Autodesk Inventor part; units mm, degrees
ref_plane "YZ Plane" through (0, 0, 0) normal (1, 0, 0) x (0, 1, 0)
ref_plane "XZ Plane" through (0, 0, 0) normal (0, 1, 0) x (-1, 0, 0)
ref_plane "XY Plane" through (0, 0, 0) normal (0, 0, 1) x (1, 0, 0)
sketch "Sketch1" plane through (0, 0, 0) normal (0, 0, 1) x (1, 0, 0)
  line L0 (68.58, 6.35) -> (68.58, 57.15)
  line L1 (68.58, 57.15) -> (0, 57.15)
  line L2 (0, 57.15) -> (0, 6.35)
  line L3 (40.64, 6.35) -> (40.64, 0)
  line L4 (27.94, 6.35) -> (27.94, 0)
  line L5 (27.94, 0) -> (40.64, 0)
  line L6 (27.94, 6.35) -> (18.8722, 6.35)
  line L7 (18.8722, 6.35) -> (18.8722, 0)
  line L8 (18.8722, 0) -> (6.1722, 0)
  line L9 (6.1722, 0) -> (6.1722, 6.35)
  line L10 (40.64, 6.35) -> (49.7078, 6.35)
  line L11 (49.7078, 6.35) -> (49.7078, 0)
  line L12 (49.7078, 0) -> (62.4078, 0)
  line L13 (62.4078, 0) -> (62.4078, 6.35)
  line L14 (6.1722, 0) -> (18.8722, 0)
  line L15 (27.94, 0) -> (40.64, 0)
  line L16 (49.7078, 0) -> (62.4078, 0)
  line L17 (27.94, 6.35) -> (18.8722, 6.35)
  line L18 (6.1722, 6.35) -> (0, 6.35)
  line L19 (40.64, 6.35) -> (49.7078, 6.35)
  line L20 (62.4078, 6.35) -> (68.58, 6.35)
  point P0 (0, 0)
  dimension "d0" = 68.58
  dimension "d1" = 50.8
extrude "Extrusion1" add sketch "Sketch1" against normal blind 6.35
sketch "Sketch2" plane through (0, 0, 0) normal (0, 0, 1) x (1, 0, 0)
  line L0 (0, 6.35) -> (6.1722, 6.35)
  line L1 (6.1722, 50.8) -> (6.1722, 57.15)
  line L2 (0, 57.15) -> (68.58, 57.15)
  line L3 (49.7078, 6.35) -> (40.64, 6.35)
  line L4 (40.64, 50.8) -> (40.64, 57.15)
  line L5 (18.8722, 0) -> (18.8722, 6.35)
  line L6 (18.8722, 50.8) -> (18.8722, 57.15)
  line L7 (27.94, 0) -> (27.94, 6.35)
  line L8 (27.94, 50.8) -> (27.94, 57.15)
  line L9 (49.7078, 50.8) -> (49.7078, 57.15)
  line L10 (68.58, 6.35) -> (62.4078, 6.35)
  line L11 (62.4078, 50.8) -> (62.4078, 57.15)
  line L12 (0, 57.15) -> (0, 50.8)
  line L13 (68.58, 57.15) -> (68.58, 6.35)
  line L14 (49.7078, 50.8) -> (62.4078, 50.8)
  line L15 (6.1722, 50.8) -> (18.8722, 50.8)
  line L16 (27.94, 50.8) -> (40.64, 50.8)
  line L17 (27.94, 57.15) -> (40.64, 57.15)
  point P0 (0, 0)
extrude "Extrusion2" cut sketch "Sketch2" against normal blind 6.35
properties part number "flat-no-recess"
Work out the finished part from the listing and answer in its coordinate system (mm). A direction names the side the tool comes from. Round coordinates to 2 decimals unless told otherwise and drop trailing zeros. Write each loop counter-clockwise with the first axis right and the second up, starting at its lowest first coordinate (ties: lowest second). Pieces come first, ordered by that corner, then holes. Notation, with made-up numbers: (75.25, 50.25) - (82.25, 50.25) arc R21 ccw to (82.25, 61.25) - close; hole circle Ø3 at (-6, -29.75). An arc over 180 degrees is marked (long way). Return JSON: item names as keys, results as strings. Group by question number.
Q1. For faces 4 (the flat face through (62.408, 54, -3)), 5 (the flat face through (27.94, 3, -3)), 6 (the flat face through (3, 6.35, -3)), determine the directions among +Z, -Z, +X, -X, +Y, -Y from which every point of the face is accessible in a straight line to the end or side of a thin tool.
Q2. The part is cut by section C-C on x = 11. Write down the section's boundary in (y, z).
Q3. The mould has two halves that part along X. Classify faces 1 (the flat face through (3, 57.15, -3)), 2 (the flat face through (68.58, 31, -3)), 3 (the flat face through (49.708, 3, -3)): released by +X, released by -X, zero draft, split by the parting line, or undercut.
Q4. Find the intervals of material crossed by L1, parallel to X at y = 54, z = -3.25; L2, parallel to X at y = 2.5, z = -1; L3, parallel to Y at x = 54, z = -5.5, in increasing order.
Q5. The part is cut by section A-A on y = 5. Write down the section's boundary in (x, z), then the cut area to 3 significant figures.
Q6. The part is cut by section B-B on z = -4.25. Write down the section's boundary in (x, y), then the cut area to 3 significant figures.
Q7. Each of these flat-tipped pins is pushed along its axis until it touches: pin 1 Ø3 at (y, z) = (3.5, -4.5) entering from +X; pin 2 Ø2 at (x, z) = (60.5, -5.5) entering from +Y; pin 3 Ø1.9 at (x, z) = (66, -4) entering from -Y. Where does it stop, or does it pass through?
Solved:
{
 "1": {"face 4": "+Z, -Z, +Y", "face 5": "+Z, -Z, -Y", "face 6": "+Z, -Z, -X, -Y"},
 "2": {"outline": "(0, -6.35) - (50.8, -6.35) - (50.8, 0) - (0, 0) - close"},
 "3": {"face 1": "zero draft", "face 2": "released by +X", "face 3": "undercut"},
 "4": {"L1": "0 to 6.17, 18.87 to 27.94, 40.64 to 49.71, 62.41 to 68.58", "L2": "6.17 to 18.87, 27.94 to 40.64, 49.71 to 62.41", "L3": "0 to 50.8"},
 "5": {"outline": "(6.17, -6.35) - (18.87, -6.35) - (18.87, 0) - (6.17, 0) - close; (27.94, -6.35) - (40.64, -6.35) - (40.64, 0) - (27.94, 0) - close; (49.71, -6.35) - (62.41, -6.35) - (62.41, 0) - (49.71, 0) - close", "area": "242 mm²"},
 "6": {"outline": "(0, 6.35) - (6.17, 6.35) - (6.17, 0) - (18.87, 0) - (18.87, 6.35) - (27.94, 6.35) - (27.94, 0) - (40.64, 0) - (40.64, 6.35) - (49.71, 6.35) - (49.71, 0) - (62.41, 0) - (62.41, 6.35) - (68.58, 6.35) - (68.58, 57.15) - (62.41, 57.15) - (62.41, 50.8) - (49.71, 50.8) - (49.71, 57.15) - (40.64, 57.15) - (40.64, 50.8) - (27.94, 50.8) - (27.94, 57.15) - (18.87, 57.15) - (18.87, 50.8) - (6.17, 50.8) - (6.17, 57.15) - (0, 57.15) - close", "area": "3,480 mm²"},
 "7": {"pin 1": "x = 62.41", "pin 2": "y = 50.8", "pin 3": "y = 6.35"}
}
